Job drawing, mm, ordinate dimensions from the low corner. One solid piece. Coordinates: 2 decimals unless noted, no trailing zeros. Order: outer loops, then holes, each group sorted by start corner. A loop starts at its lowest first (then second) coordinate and runs counter-clockwise, first axis right, second up. Notation, with made-up numbers: (-32, 58.25) - (-19, 58.25) arc R35 cw to (-19, 97.25) - close; hole circle Ø11 at (73.5, 15.5). An arc over 180 degrees is marked (long way). Use a Markdown table: item, result. Add a question column.
1) Two-plate mould, pull along X, no slides. Class the marked faces 1, 2 and 3: +X half, -X half, draft (parallel to the pull), parting line (faces both ways), or undercut.
2) Wall check: L1, parallel to X at y = 3, z = 0.7 (1 decimal); L2, parallel to X at y = 5.75, z = 1.9 (1 decimal); L3, parallel to Y at x = 1.25, z = 1.3. Give the ranges that are in metal, low to high. Write a range as [from, to].
3) Saw through at A-A on x = 4.25. List the corners of the cut face in (y, z).
4) Saw through at D-D on y = 1.5. List the corners of the cut face in (x, z).
5) Drop a flat-ended pin along its axis: P1, Ø1.5, axis at y = 1, z = 1.5, coming from the -X side. Give the stop position or say it passes through.
6) Saw through at B-B on y = 6. List the corners of the cut face in (x, z), then the cut area to 3 significant figures.
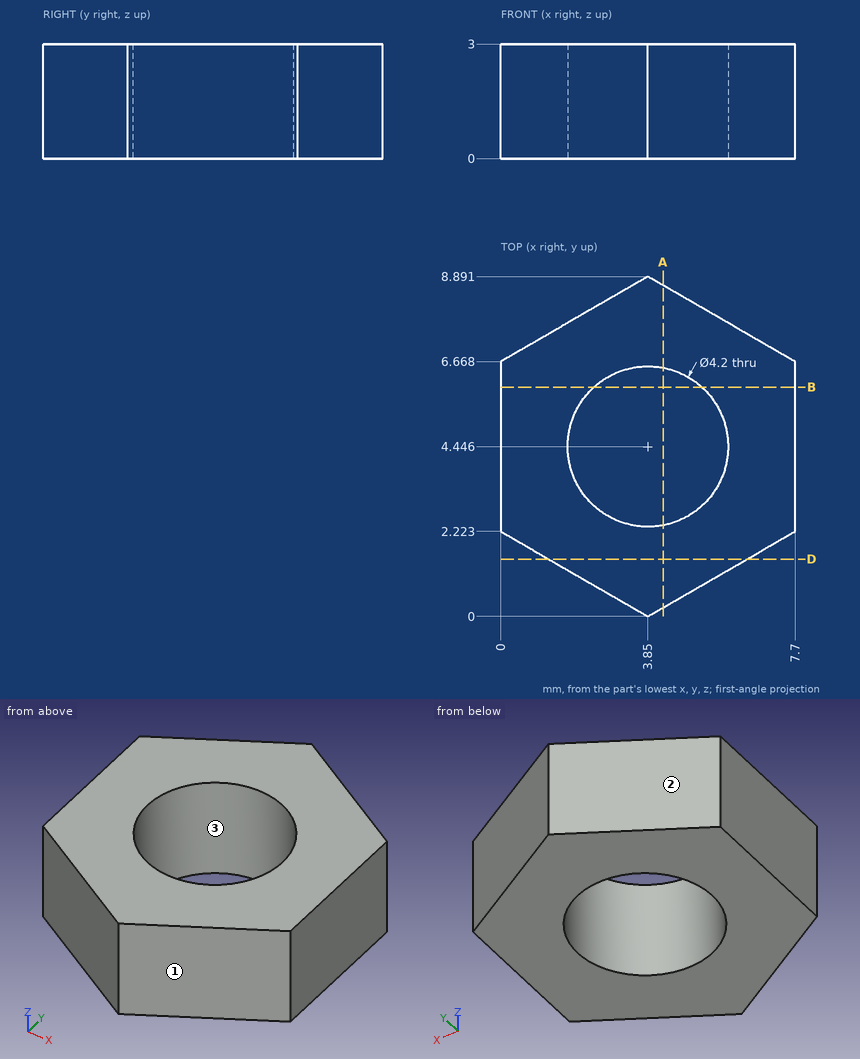
Results are:
| question | item | result |
|---|---|---|
| 1 | face 1 | +X half |
| 1 | face 2 | -X half |
| 1 | face 3 | undercut |
| 2 | L1 | [0, 2.3], [5.4, 7.7] |
| 2 | L2 | [0, 2.2], [5.5, 7.7] |
| 2 | L3 | [1.5, 7.39] |
| 3 | outline | (0.23, 0) - (2.38, 0) - (2.38, 3) - (0.23, 3) - close; (6.51, 0) - (8.66, 0) - (8.66, 3) - (6.51, 3) - close |
| 4 | outline | (1.25, 0) - (6.45, 0) - (6.45, 3) - (1.25, 3) - close |
| 5 | P1 | x = 0.82 |
| 6 | outline | (0, 0) - (2.44, 0) - (2.44, 3) - (0, 3) - close; (5.26, 0) - (7.7, 0) - (7.7, 3) - (5.26, 3) - close |
| 6 | area | 14.6 mm2 |
